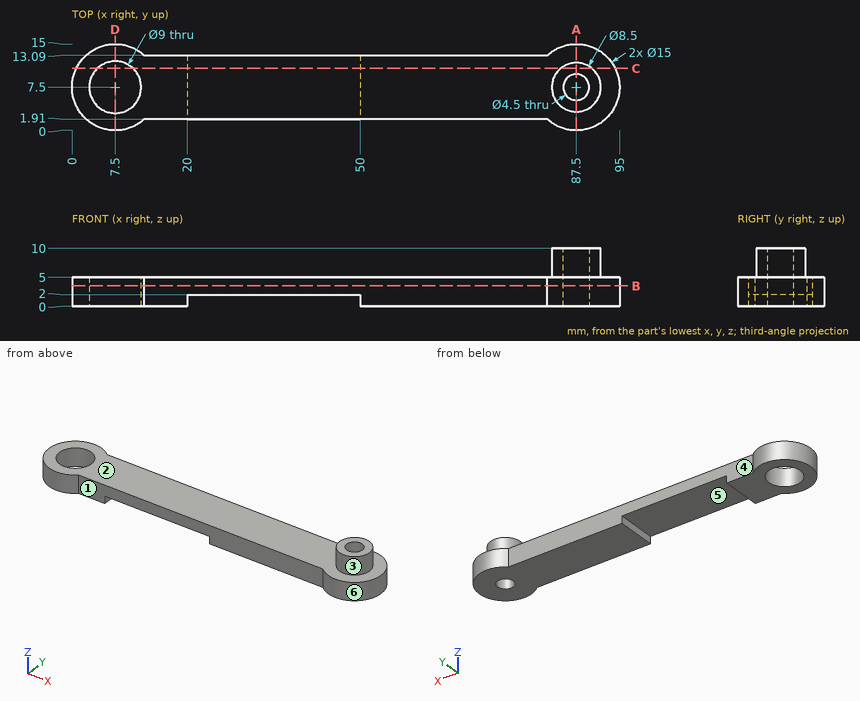
Design review of the part shown in the three views and the two pictorial views. Dimensions are in mm from the part's minimum x, y and z. A direction names the side the tool comes from. Round coordinates to 2 decimals unless told otherwise and drop trailing zeros. Write each loop counter-clockwise with the first axis right and the second up, starting at its lowest first coordinate (ties: lowest second). Pieces come first, ordered by that corner, then holes. Notation, with made-up numbers: M 11.25,-15.5 L 53.25,-15.5 A23 ccw 53.25,22.5 Z; hole C 42.5,77.25 d8. An arc over 180 degrees is marked long. One line per item, written item: value. Start each with the question number.
1. To check wall thickness, follow probe 1 along Y at (x, z) = (7.5, 3.35); probe 2 along Z at (x, y) = (31, 8); probe 3 along Z at (x, y) = (73, 10). State the ranges of each line that lie inside material, in increasing order. Write a range as from..to.
2. Clearance check with flat-ended pins moving along their axes: P1, Ø7.5, axis at x = 71, y = 10.5, coming from the +Z side; P2, Ø2.5, axis at x = 41.5, z = 1.5, coming from the +Y side; P3, Ø1.6, axis at y = 6, z = 0.5, coming from the +X side. State where each tip first meets the part, or that it passes through.
3. Take a section at A-A on x = 87.5. State the section outline as (y, z) points, then the cut area to 3 significant figures.
4. Draft analysis for pull direction X (two halves, no side actions). For the marked faces 1, 2 and 3, state which applies: pulls with the +X half, pulls with the -X half, needs draft (parallel to the pull), parting line crosses it, or undercut.
5. Take a section at B-B on z = 3.5. State the section outline as (x, y) points, then the cut area to 3 significant figures.
6. For the marked faces 4, 5 and 6, list the 3-axis set-ups (+Z, -Z, +X, -X, +Y, -Y) from which the entire face can be reached by the end or side of a thin tool; tool diameter is ignored.
7. Take a section at C-C on y = 10.75. State the section outline as (x, z) points.
8. Take a section at D-D on x = 7.5. State the section outline as (y, z) points.
Computed:
1. probe 1: y = 0..3, 12..15
1. probe 2: z = 2..5
1. probe 3: z = 0..5
2. P1: stops at z = 5
2. P2: stops at y = 13.09
2. P3: stops at x = 94.97
3. outline: M 0,0 L 5.25,0 L 5.25,10 L 3.25,10 L 3.25,5 L 0,5 Z; M 9.75,0 L 15,0 L 15,5 L 11.75,5 L 11.75,10 L 9.75,10 Z
3. area: 72.5 mm²
4. face 1: undercut
4. face 2: needs draft
4. face 3: parting line crosses it
5. outline: M 12.5,1.91 L 82.5,1.91 A7.5 ccw long 82.5,13.09 L 12.5,13.09 A7.5 ccw long Z; hole C 7.5,7.5 d9; hole C 87.5,7.5 d4.5
5. area: 1,020 mm²
6. face 4: +Z, -Z, +Y
6. face 5: -Z, +Y, -Y
6. face 6: +Z, -Z
7. outline: M 0.74,0 L 4.39,0 L 4.39,5 L 0.74,5 Z; M 10.61,0 L 20,0 L 20,2 L 50,2 L 50,0 L 94.26,0 L 94.26,5 L 90.24,5 L 90.24,10 L 84.76,10 L 84.76,5 L 10.61,5 Z
8. outline: M 0,0 L 3,0 L 3,5 L 0,5 Z; M 12,0 L 15,0 L 15,5 L 12,5 Z
